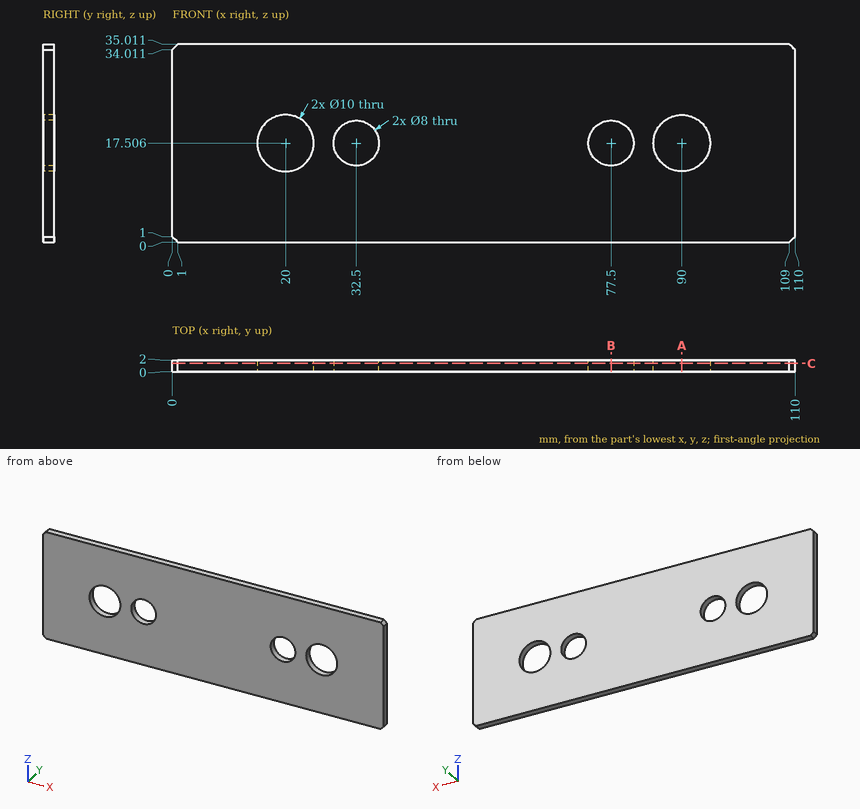
Here's the drawing with two shaded views (mm, measured from the low corner). I have some questions. Round coordinates to 2 decimals unless told otherwise and drop trailing zeros. Order: outer loops, then holes, each group sorted by start corner. A loop starts at its lowest first (then second) coordinate and runs counter-clockwise, first axis right, second up. Notation, with made-up numbers: (65.25, -34) -> (78.25, -34) arc R23 cw to (78.25, 2) -> close; hole circle Ø9 at (43, 45). An arc over 180 degrees is marked (long way). Write each question's results on one line, items separated by ' | '. Start each with the question number.
Item 1: If we section it at A-A, the plane x = 90: Write out the boundary of the cut face in (y, z) (1 decimal).
Item 2: Will this pin go through, and if not, where does the flat tip stop? pin 1 (8 mm diameter, centred on x = 20, z = 17.51, fed in from -Y).
Item 3: Please list where these lines run through material, in increasing order: L1, parallel to Z at x = 77.5, y = 1.15 (1 decimal); L2, parallel to Z at x = 90, y = 1.1 (1 decimal); L3, parallel to X at y = 1.35, z = 19.
Item 4: If we section it at B-B, the plane x = 77.5: Write out the boundary of the cut face in (y, z) (1 decimal).
Item 5: If we section it at C-C, the plane y = 1.45: Write out the boundary of the cut face in (x, z) (1 decimal).
Results:
1) outline: (0, 0) -> (2, 0) -> (2, 12.5) -> (0, 12.5) -> close; (0, 22.5) -> (2, 22.5) -> (2, 35) -> (0, 35) -> close
2) pin 1: passes through
3) L1: z = 0 to 13.5, 21.5 to 35 | L2: z = 0 to 12.5, 22.5 to 35 | L3: x = 0 to 15.23, 24.77 to 28.79, 36.21 to 73.79, 81.21 to 85.23, 94.77 to 110
4) outline: (0, 0) -> (2, 0) -> (2, 13.5) -> (0, 13.5) -> close; (0, 21.5) -> (2, 21.5) -> (2, 35) -> (0, 35) -> close
5) outline: (0, 1) -> (1, 0) -> (109, 0) -> (110, 1) -> (110, 34) -> (109, 35) -> (1, 35) -> (0, 34) -> close; hole circle Ø10 at (20, 17.5); hole circle Ø8 at (32.5, 17.5); hole circle Ø8 at (77.5, 17.5); hole circle Ø10 at (90, 17.5)
